Input: part model. Units: mm. Frame: model coordinates. A direction names the side the tool comes from. Round coordinates to 2 decimals unless told otherwise and drop trailing zeros. Loops run counter-clockwise (first coordinate to the right, second up) from the corner with the lowest first, then second, coordinate; pieces in that order, holes last.
1) Draft query along Z for faces 4 (the face through (-17.564, 6.482, -34.185)), 5 (the face through (0, 0, 50.8)), 6 (the face through (18.46, -3.81, 32.17)), 7 (the face through (-1, -16.51, -1)). Return one class per face: pulls with the +Z half, pulls with the -Z half, needs draft (parallel to the pull), parting line crosses it, or undercut.
2) Section D-D, the plane x = 48.5. Return loops of the section in (y, z).
3) Ray query, line 1 along X through (y, z) = (8, 0); line 2 along X through (y, z) = (8, -31.75); line 3 along X through (y, z) = (4.5, 25). Return the intervals inside material, ascending.
4) Section C-C, the plane z = 42. Return loops of the section in (x, y).
5) Access query for faces 1 (the face through (-17.564, 6.482, 29.315)), 2 (the face through (-26.2, 0.2, -15.6)), 3 (the face through (-44.2, 3.9, 25.04)). Directions: +Z, -Z, +X, -X, +Y, -Y. A direction counts if a zero-diameter tool reaches every point of the face in a straight line with its end or side. Return the directions, or none.
6) Section B-B, the plane y = 9.5. Return loops of the section in (x, z).
7) Section A-A, the plane y = -6.5. Return loops of the section in (x, z), and give its area (3 significant figures).
8) First-contact query: pin 1 (6.5 mm diameter, centred on x = -18.33, z = 31.75, fed in from +Y); pin 2 (12 mm diameter, centred on y = -3, z = -13, fed in from -X); pin 3 (4 mm diameter, centred on x = -18.33, z = -31.75, fed in from +Y). Flat tips, straight axial feed; report the tip coordinate or a pass-through.
from build123d import *

# Parameters (mm, degrees)
BOSS_EXTRUDE1_DEPTH                         = 16.51
F_1_4_20_TAPPED_HOLE1_D                     = 5.1054
F_1_4_20_TAPPED_HOLE1_DEPTH                 = 19.05
F_1_4_20_TAPPED_HOLE1_CSINK_D               = 6.604
F_1_4_20_TAPPED_HOLE1_CSINK_ANGLE           = 90
F_1_4_20_TAPPED_HOLE1_TIP                   = 1.533816902
F_1_4_20_TAPPED_HOLE1_ON_FACE_2_D           = 5.1054
F_1_4_20_TAPPED_HOLE1_ON_FACE_2_DEPTH       = 19.05
F_1_4_20_TAPPED_HOLE1_ON_FACE_2_CSINK_D     = 6.604
F_1_4_20_TAPPED_HOLE1_ON_FACE_2_CSINK_ANGLE = 90
F_1_4_20_TAPPED_HOLE1_ON_FACE_2_TIP         = 1.533816902
F_1_4_20_TAPPED_HOLE1_ON_FACE_3_D           = 5.1054
F_1_4_20_TAPPED_HOLE1_ON_FACE_3_DEPTH       = 19.05
F_1_4_20_TAPPED_HOLE1_ON_FACE_3_CSINK_D     = 6.604
F_1_4_20_TAPPED_HOLE1_ON_FACE_3_CSINK_ANGLE = 90
F_1_4_20_TAPPED_HOLE1_ON_FACE_3_TIP         = 1.533816902


with BuildPart() as part:
    # Sketch1 → Boss-Extrude1 (new, symmetric)
    with BuildSketch(Plane(origin=(0, 0, 0), x_dir=(1, 0, 0), z_dir=(0, 1, 0))):
        Polygon((-58.65878735, 0), (-29.329393675, -50.8), (29.329393675, -50.8), (58.65878735, 0), (29.329393675, 50.8), (-29.329393675, 50.8), align=None)
    extrude(amount=BOSS_EXTRUDE1_DEPTH, both=True)

    # 1/4-20 Tapped Hole1
    with Locations(Plane(origin=(-43.994090512, 0, -25.4), x_dir=(0.5, 0, -0.866025403784), z_dir=(-0.866025403784, 0, -0.5))):
        with Locations((0, 0)):
            CounterSinkHole(F_1_4_20_TAPPED_HOLE1_D / 2, F_1_4_20_TAPPED_HOLE1_CSINK_D / 2, depth=F_1_4_20_TAPPED_HOLE1_DEPTH, counter_sink_angle=F_1_4_20_TAPPED_HOLE1_CSINK_ANGLE)
            with Locations((0, 0, -(F_1_4_20_TAPPED_HOLE1_DEPTH + F_1_4_20_TAPPED_HOLE1_TIP / 2))):  # 118° drill point
                Cone(0, F_1_4_20_TAPPED_HOLE1_D / 2, F_1_4_20_TAPPED_HOLE1_TIP, mode=Mode.SUBTRACT)

    # 1/4-20 Tapped Hole1 on face 2
    with Locations(Plane(origin=(-43.994090512, 0, 25.4), x_dir=(-0.500000174844, 0, -0.866025302838), z_dir=(-0.866025302838, 0, 0.500000174844))):
        with Locations((0, 0)):
            CounterSinkHole(F_1_4_20_TAPPED_HOLE1_ON_FACE_2_D / 2, F_1_4_20_TAPPED_HOLE1_ON_FACE_2_CSINK_D / 2, depth=F_1_4_20_TAPPED_HOLE1_ON_FACE_2_DEPTH, counter_sink_angle=F_1_4_20_TAPPED_HOLE1_ON_FACE_2_CSINK_ANGLE)
            with Locations((0, 0, -(F_1_4_20_TAPPED_HOLE1_ON_FACE_2_DEPTH + F_1_4_20_TAPPED_HOLE1_ON_FACE_2_TIP / 2))):  # 118° drill point
                Cone(0, F_1_4_20_TAPPED_HOLE1_ON_FACE_2_D / 2, F_1_4_20_TAPPED_HOLE1_ON_FACE_2_TIP, mode=Mode.SUBTRACT)

    # 1/4-20 Tapped Hole1 on face 3
    with Locations(Plane(origin=(18.330871047, 16.51, 31.75), x_dir=(0, 0, 1), z_dir=(0, 1, 0))):
        with Locations((0, 0), (-31.75, 18.330871047), (-63.5, -36.661742094), (-31.75, -54.992613141), (0, -36.661742094), (-63.5, 0)):
            CounterSinkHole(F_1_4_20_TAPPED_HOLE1_ON_FACE_3_D / 2, F_1_4_20_TAPPED_HOLE1_ON_FACE_3_CSINK_D / 2, depth=F_1_4_20_TAPPED_HOLE1_ON_FACE_3_DEPTH, counter_sink_angle=F_1_4_20_TAPPED_HOLE1_ON_FACE_3_CSINK_ANGLE)
            with Locations((0, 0, -(F_1_4_20_TAPPED_HOLE1_ON_FACE_3_DEPTH + F_1_4_20_TAPPED_HOLE1_ON_FACE_3_TIP / 2))):  # 118° drill point
                Cone(0, F_1_4_20_TAPPED_HOLE1_ON_FACE_3_D / 2, F_1_4_20_TAPPED_HOLE1_ON_FACE_3_TIP, mode=Mode.SUBTRACT)


solid = part.part
Final values:
1. face 4: undercut
1. face 5: pulls with the +Z half
1. face 6: undercut
1. face 7: needs draft
2. outline: (-16.51, -17.6) - (16.51, -17.6) - (16.51, 17.6) - (-16.51, 17.6) - close
3. line 1: x = -58.66 to -39.21, -34.11 to 34.11, 39.21 to 58.66
3. line 2: x = -40.33 to -20.88, -15.78 to 15.78, 20.88 to 40.33
3. line 3: x = -44.23 to 44.23
4. outline: (-34.41, -16.51) - (34.41, -16.51) - (34.41, 16.51) - (-34.41, 16.51) - close
5. face 1: +Y
5. face 2: none
5. face 3: +Z, -X, +Y, -Y
6. outline: (-58.66, 0) - (-29.33, -50.8) - (29.33, -50.8) - (58.66, 0) - (29.33, 50.8) - (-29.33, 50.8) - close; hole circle Ø5.11 at (-36.66, 0); hole circle Ø5.11 at (-18.33, -31.75); hole circle Ø5.11 at (-18.33, 31.75); hole circle Ø5.11 at (18.33, -31.75); hole circle Ø5.11 at (18.33, 31.75); hole circle Ø5.11 at (36.66, 0)
7. outline: (-58.66, 0) - (-29.33, -50.8) - (29.33, -50.8) - (58.66, 0) - (29.33, 50.8) - (-29.33, 50.8) - close
7. area: 8,940 mm2
8. pin 1: stops at y = 16.46
8. pin 2: stops at x = -54.62
8. pin 3: stops at y = -2.87
